Autodesk Inventor part; units mm, degrees
ref_plane "YZ Plane" through (0, 0, 0) normal (1, 0, 0) x (0, 1, 0)
ref_plane "XZ Plane" through (0, 0, 0) normal (0, 1, 0) x (-1, 0, 0)
ref_plane "XY Plane" through (0, 0, 0) normal (0, 0, 1) x (1, 0, 0)
sketch "草图1" plane through (0, 0, 0) normal (0, 1, 0) x (-1, 0, 0)
  line L0 (40, 40) -> (-40, 40)
  line L1 (-40, 40) -> (-40, -40)
  line L2 (-40, -40) -> (40, -40)
  line L3 (40, -40) -> (40, 40)
  point P0 (0, 0)
  dimension "d13" = 80
  dimension "d14" = 80
extrude "拉伸1" add sketch "草图1" along normal blind 10
fillet "圆角1" radius 2 12 edges at (-40, 5, -40) (-40, 5, 40) (-40, 0, 0) (-40, 10, 0) (40, 5, -40) (0, 0, -40) (0, 10, -40) (40, 5, 40) (40, 0, 0) (40, 10, 0) (0, 0, 40) (0, 10, 40)
sketch "草图4" plane through (0, 0, 0) normal (0, -1, 0) x (1, 0, 0)
  circle A0 centre (-35, -20) radius 2
  point P0 (0, 0)
  dimension "d15" = 4
extrude "拉伸4" cut sketch "草图4" against normal through all
sketch "草图5" plane through (0, 0, 0) normal (0, -1, 0) x (1, 0, 0)
  circle A0 centre (-35, 10) radius 2
  point P0 (0, 0)
  dimension "d18" = 4
extrude "拉伸5" cut sketch "草图5" against normal through all
properties part number "升降板"
Model file for the job. Use its own axes, mm. Coordinates: 2 decimals unless noted, no trailing zeros. Order: outer loops, then holes, each group sorted by start corner. A loop starts at its lowest first (then second) coordinate and runs counter-clockwise, first axis right, second up. Notation, with made-up numbers: (65.25, 79) -> (120.25, 79) arc R18 cw to (120.25, 112) -> close; hole circle Ø8 at (6.25, 36). An arc over 180 degrees is marked (long way). Return JSON: item names as keys, results as strings. Group by question number.
Item 1: Pull direction X, two halves, no side cores. Call faces 1 (the cylindrical face through (-35, 5, -18)), 2 (the cylindrical face through (0.53, 0.6, 39.43)), 3 (the cylindrical face through (-39.43, 5.04, 39.4)): pulls with the +X half, pulls with the -X half, needs draft (parallel to the pull), parting line crosses it, or undercut.
Item 2: Wall check: line 1 along Z through (x, y) = (-35, 4.75); line 2 along X through (y, z) = (8.25, 21.5); line 3 along X through (y, z) = (9.25, 11). Give the ranges that are in metal, low to high. Write a range as [from, to].
Item 3: Saw through at B-B on z = -20. Write the cut outline in (x, y).
Item 4: Saw through at C-C on y = 9. Write the cut outline in (x, z).
Item 5: Flat gauge pin, fed straight in: P1, Ø3.5, axis at x = -35, z = -20, coming from the -Y side. Where does the tip first touch, or does it go through?
Item 6: Saw through at A-A on x = -35. Write the cut outline in (y, z), then the cut area to 3 significant figures.
Values found:
{
 "1": {"face 1": "undercut", "face 2": "needs draft", "face 3": "pulls with the -X half"},
 "2": {"line 1": "z = [-40, -22], [-18, 8], [12, 40]", "line 2": "x = [-39.98, 39.98]", "line 3": "x = [-39.56, -36.73], [-33.27, 39.56]"},
 "3": {"outline": "(-40, 2) arc R2 ccw to (-38, 0) -> (-37, 0) -> (-37, 10) -> (-38, 10) arc R2 ccw to (-40, 8) -> close; (-33, 0) -> (38, 0) arc R2 ccw to (40, 2) -> (40, 8) arc R2 ccw to (38, 10) -> (-33, 10) -> close"},
 "4": {"outline": "(-39.73, -38) arc R1.73 ccw to (-38, -39.73) -> (38, -39.73) arc R1.73 ccw to (39.73, -38) -> (39.73, 38) arc R1.73 ccw to (38, 39.73) -> (-38, 39.73) arc R1.73 ccw to (-39.73, 38) -> close; hole circle Ø4 at (-35, -20); hole circle Ø4 at (-35, 10)"},
 "5": {"P1": "passes through"},
 "6": {"outline": "(0, -38) arc R2 ccw to (2, -40) -> (8, -40) arc R2 ccw to (10, -38) -> (10, -22) -> (0, -22) -> close; (0, -18) -> (10, -18) -> (10, 8) -> (0, 8) -> close; (0, 12) -> (10, 12) -> (10, 38) arc R2 ccw to (8, 40) -> (2, 40) arc R2 ccw to (0, 38) -> close", "area": "717 mm2"}
}
